from build123d import *

# Parameters (mm, degrees)
F0_W      = 160
F0_H      = 160
F1_DEPTH  = 15
F2_R      = 15
F3_DEPTH  = 25
F4_R      = 17.5
F5_DEPTH  = 10
F6_R      = 10
F7_W      = 60
F7_H      = 70
F8_DEPTH  = 7
F9_R      = 19.125
F10_DEPTH = 25
F11_R     = 3.25
F12_DEPTH = 25
F13_R     = 3.25
F14_DEPTH = 25


with BuildPart() as f1:
    # F0 (on Front) → F1 (new body)
    with BuildSketch(Plane.XZ):
        Rectangle(F0_W, F0_H)
    extrude(amount=F1_DEPTH)

    # F2 (on face) → F3 (cut)
    with BuildSketch(Plane.XZ.offset(15)):
        Circle(F2_R)
    extrude(amount=-F3_DEPTH, mode=Mode.SUBTRACT)

    # F4 (on face) → F5 (cut)
    with BuildSketch(Plane.XZ.offset(15)):
        Circle(F4_R)
    extrude(amount=-F5_DEPTH, mode=Mode.SUBTRACT)

    # F6
    f6_edges = [f1.edges().sort_by_distance(p)[0] for p in [
        (80, -7.5, 80),
        (80, -7.5, -80),
        (-80, -7.5, -80),
        (-80, -7.5, 80),
    ]]
    fillet(f6_edges, radius=F6_R)

    # F7 (on face) → F8 (cut)
    with BuildSketch(Plane.XZ.offset(15)):
        with Locations((50, 0)):
            Rectangle(F7_W, F7_H)
    extrude(amount=-F8_DEPTH, mode=Mode.SUBTRACT)

    # F9 (on face) → F10 (cut)
    with BuildSketch(Plane(origin=(0, 0, 0), x_dir=(-1, 0, 0), z_dir=(0, 1, 0))):
        with Locations((-50, 0)):
            Circle(F9_R)
    extrude(amount=-F10_DEPTH, mode=Mode.SUBTRACT)

    # F11 (on face) → F12 (cut)
    with BuildSketch(Plane.XZ.offset(8)):
        with Locations((26.45, 23.55)):
            Circle(F11_R)
        with Locations((26.45, -23.55)):
            Circle(F11_R)
        with Locations((73.55, -23.55)):
            Circle(F11_R)
        with Locations((73.55, 23.55)):
            Circle(F11_R)
    extrude(amount=-F12_DEPTH, mode=Mode.SUBTRACT)

    # F13 (on face) → F14 (cut)
    with BuildSketch(Plane.XZ.offset(15)):
        with Locations((70, 70)):
            Circle(F13_R)
        with Locations((-70, 70)):
            Circle(F13_R)
        with Locations((-70, -70)):
            Circle(F13_R)
        with Locations((70, -70)):
            Circle(F13_R)
    extrude(amount=-F14_DEPTH, mode=Mode.SUBTRACT)


solid = f1.part
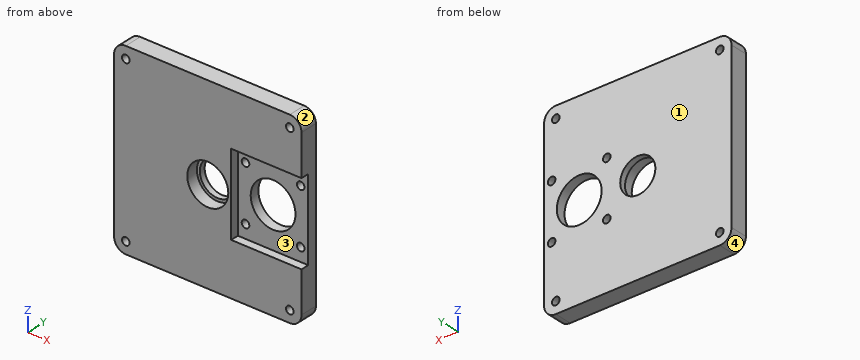
Could you check a few things on this model? Use its own coordinates, in mm. Face numbers are marked on the shaded views. Coordinates: 2 decimals unless noted, no trailing zeros. Write each loop counter-clockwise with the first axis right and the second up, starting at its lowest first coordinate (ties: lowest second). Pieces come first, ordered by that corner, then holes. Notation, with made-up numbers: (52, 53.5) - (104, 53.5) arc R16 ccw to (104, 73.5) - close; hole circle Ø6 at (52.5, -9). An arc over 180 degrees is marked (long way). Put each result on its own line as item: value. Start each with the question number.
Q1. I want a section at C-C on x = 26.45. Write out the boundary of the cut face in (y, z), plus the area to 3 significant figures.
Q2. Please list where these lines run through material, in increasing order: L1, parallel to Z at x = 26.45, y = -3.25; L2, parallel to Z at x = 70, y = -6.5; L3, parallel to Z at x = 50, y = -2.25 (3 decimals).
Q3. I want a section at B-B on z = 0. Write out the boundary of the cut face in (x, y) (3 decimals).
Q4. Thinking about a two-plate mould opening in Z: for the marked faces 1, 2, 3 and 4, which applies, pulls with the +Z half, pulls with the -Z half, needs draft (parallel to the pull), parting line crosses it, or undercut?
Q5. I want a section at D-D on y = -11.5. Write out the boundary of the cut face in (x, z), plus the area to 3 significant figures.
Q6. I'm going to push flat-ended pins straight in: P1, Ø8.5, axis at x = 26.45, z = 23.55, coming from the -Y side; P2, Ø5, axis at x = 73.55, z = 23.55, coming from the -Y side; P3, Ø3.5, axis at y = -11.5, z = 1.5, coming from the +X side. Where does each tip first touch, or does it pass through?
Q7. I want a section at A-A on x = 0. Write out the boundary of the cut face in (y, z), plus the area to 3 significant figures.
Checks:
1. outline: (-15, -80) - (0, -80) - (0, -26.8) - (-8, -26.8) - (-8, -35) - (-15, -35) - close; (-15, 35) - (-8, 35) - (-8, 26.8) - (0, 26.8) - (0, 80) - (-15, 80) - close; (-8, -20.3) - (0, -20.3) - (0, 20.3) - (-8, 20.3) - close
1. area: 1,810 mm²
2. L1: -80 to -26.8, -20.3 to 20.3, 26.8 to 80
2. L2: -80 to -73.25, -66.75 to 66.75, 73.25 to 80
2. L3: -80 to -19.125, 19.125 to 80
3. outline: (-80, -15) - (-17.5, -15) - (-17.5, -5) - (-15, -5) - (-15, 0) - (-80, 0) - close; (15, -5) - (17.5, -5) - (17.5, -15) - (20, -15) - (20, -8) - (30.875, -8) - (30.875, 0) - (15, 0) - close; (69.125, -8) - (80, -8) - (80, 0) - (69.125, 0) - close
4. face 1: needs draft
4. face 2: pulls with the +Z half
4. face 3: undercut
4. face 4: pulls with the -Z half
5. outline: (-80, -70) arc R10 ccw to (-70, -80) - (70, -80) arc R10 ccw to (80, -70) - (80, -35) - (20, -35) - (20, 35) - (80, 35) - (80, 70) arc R10 ccw to (70, 80) - (-70, 80) arc R10 ccw to (-80, 70) - close; hole circle Ø6.5 at (-70, -70); hole circle Ø6.5 at (-70, 70); hole circle Ø35 at (0, 0); hole circle Ø6.5 at (70, -70); hole circle Ø6.5 at (70, 70)
5. area: 20,200 mm²
6. P1: y = -8
6. P2: through
6. P3: x = 20
7. outline: (-15, -80) - (0, -80) - (0, -15) - (-5, -15) - (-5, -17.5) - (-15, -17.5) - close; (-15, 17.5) - (-5, 17.5) - (-5, 15) - (0, 15) - (0, 80) - (-15, 80) - close
7. area: 1,900 mm²
